Build history of the part. All positions in model axes, mm. Coordinates: 2 decimals unless noted, no trailing zeros. Write each loop counter-clockwise with the first axis right and the second up, starting at its lowest first coordinate (ties: lowest second). Pieces come first, ordered by that corner, then holes. Notation, with made-up numbers: (-4, -10) -> (10, -10) arc R23 ccw to (10, 12) -> close; hole circle Ø10 at (18.25, -5). An arc over 180 degrees is marked (long way). Write each question's results on one line, items separated by ' | '. Start each with the question number.
Q1. Drill centre lines: line 1 (Z direction, x = 1.75, y = 23); line 2 (Y direction, x = 1.2, z = 89.5); line 3 (Y direction, x = 1.75, z = 79). Where is each one in solid material? Low to high.
Q2. Saw through at B-B on y = 23. Give the cut face in (x, z).
Q3. Saw through at C-C on x = 0.8. Give the cut face in (y, z).
Q4. Drop flat-ended pins along their axis: pin 1 Ø1 at (x, z) = (1, 24.5) entering from -Y; pin 2 Ø2.5 at (y, z) = (18.33, 96.15) entering from +X; pin 3 Ø0.6 at (x, z) = (1, 29) entering from +Y. Give the stop position or say it passes through.
Autodesk Inventor part; units mm, degrees
ref_plane "YZ Plane" through (0, 0, 0) normal (1, 0, 0) x (0, 1, 0)
ref_plane "XZ Plane" through (0, 0, 0) normal (0, 1, 0) x (-1, 0, 0)
ref_plane "XY Plane" through (0, 0, 0) normal (0, 0, 1) x (1, 0, 0)
sketch "Szkic1" plane through (0, 0, 0) normal (1, 0, 0) x (0, 1, 0)
  circle A0 centre (18.3256, 3.8503) radius 1.5
  circle A1 centre (18.3256, 96.1497) radius 1.5
  line L0 (15.3555, 36.8868) -> (29.2091, 36.8868)
  line L1 (29.2091, 36.8868) -> (29.2091, 7.7086)
  line L2 (29.2091, 7.7086) -> (15.3555, 7.7086)
  line L3 (15.3555, 7.7086) -> (15.3555, 36.8868)
  line L4 (15.3555, 92.2914) -> (29.2091, 92.2914)
  line L5 (29.2091, 92.2914) -> (29.2091, 63.1132)
  line L6 (29.2091, 63.1132) -> (15.3555, 63.1132)
  line L7 (15.3555, 63.1132) -> (15.3555, 92.2914)
  line L8 (0, 100) -> (43.598, 100)
  line L9 (0, 100) -> (0, 0)
  line L10 (43.598, 0) -> (0, 0)
  line L11 (43.598, 100) -> (43.598, 0)
  line L12 (43.598, 100) -> (44.6676, 100)
  line L13 (43.598, 100) -> (43.598, 0)
  line L14 (44.6676, 0) -> (43.598, 0)
  line L15 (44.6676, 100) -> (44.6676, 0)
  point P0 (33.9001, 100)
extrude "Wyciągnięcie proste1" add sketch "Szkic1" along normal blind 2
chamfer "Faza1" distance 2 angle 45 1 edges at (2, 44.6676, 50)
chamfer "Faza2" distance 2 angle 45 1 edges at (0, 0, 50)
properties part number "kopia_plug"
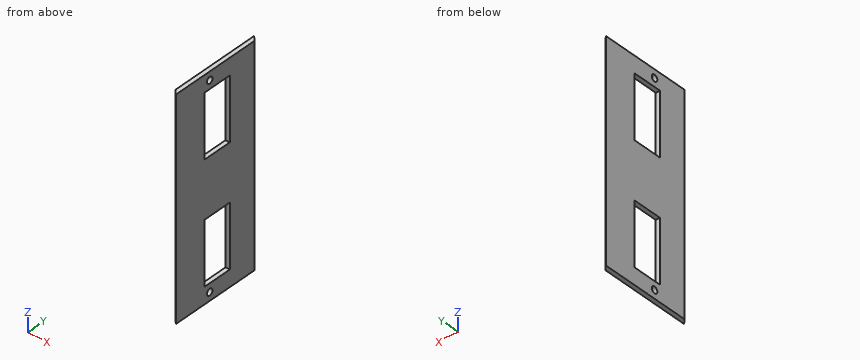
Returned:
1) line 1: z = 0 to 7.71, 36.89 to 63.11, 92.29 to 100 | line 2: y = 0.8 to 15.36, 29.21 to 43.47 | line 3: y = 0.25 to 15.36, 29.21 to 42.92
2) outline: (0, 0) -> (2, 0) -> (2, 7.71) -> (0, 7.71) -> close; (0, 36.89) -> (2, 36.89) -> (2, 63.11) -> (0, 63.11) -> close; (0, 92.29) -> (2, 92.29) -> (2, 100) -> (0, 100) -> close
3) outline: (1.2, 0) -> (43.87, 0) -> (43.87, 100) -> (1.2, 100) -> close; hole (15.36, 7.71) -> (29.21, 7.71) -> (29.21, 36.89) -> (15.36, 36.89) -> close; hole (15.36, 63.11) -> (29.21, 63.11) -> (29.21, 92.29) -> (15.36, 92.29) -> close; hole circle Ø3 at (18.33, 3.85); hole circle Ø3 at (18.33, 96.15)
4) pin 1: stops at y = 0.5 | pin 2: passes through | pin 3: stops at y = 43.97
